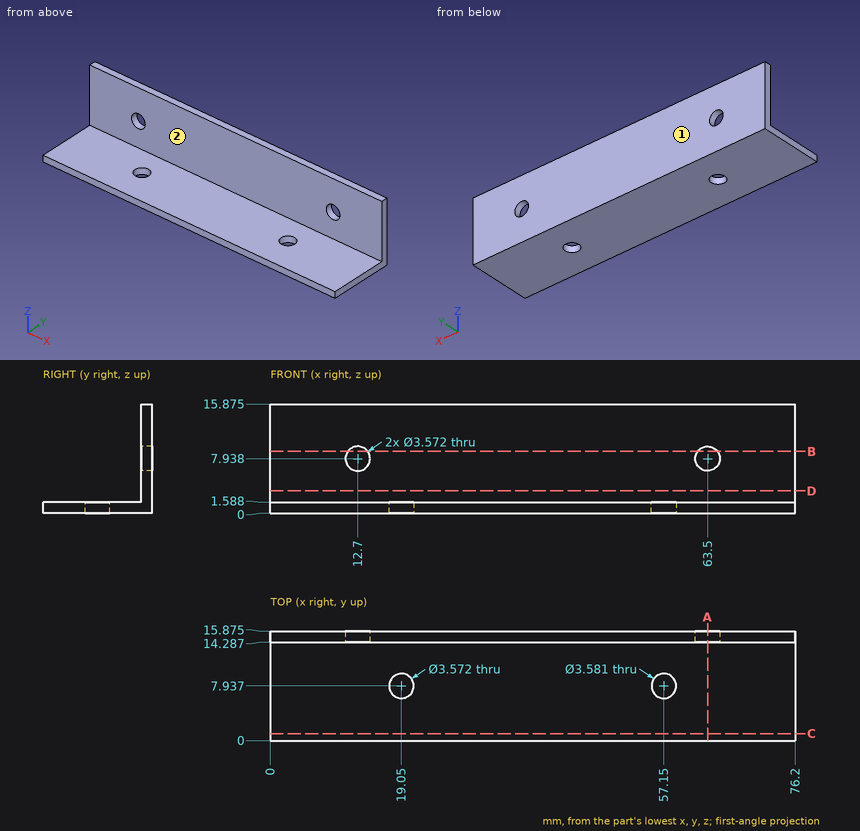
Check sheet for the drawn part. Datum: minimum x, y, z corner. Units: mm. A direction names the side the tool comes from. Coordinates: 2 decimals unless noted, no trailing zeros. Order: outer loops, then holes, each group sorted by start corner. A loop starts at its lowest first (then second) coordinate and runs counter-clockwise, first axis right, second up. Notation, with made-up numbers: M 55.25,-10.75 L 74.25,-10.75 A19 ccw 74.25,10.25 Z; hole C -20,12 d5. An arc over 180 degrees is marked long. One line per item, written item: value. Start each with the question number.
Item 1: Gauge pin test, flat ends, axial feed: pin 1 (1 mm diameter, centred on y = 10.5, z = 3, fed in from -X); pin 2 (8 mm diameter, centred on x = 46, y = 8.5, fed in from -Z); pin 3 (5.5 mm diameter, centred on x = 57.15, y = 7.94, fed in from +Z); pin 4 (4 mm diameter, centred on x = 12.7, z = 7.94, fed in from -Y). Record the tip position at first contact, or that the pin passes through.
Item 2: Access from +Z, -Z, +X, -X, +Y, -Y to the whole of each face (thin tool, end or side, straight path). Record for the marked faces 1 and 2.
Item 3: Sectioned sample at D-D (z = 3.25). Enter the section's corners in (x, y) (1 decimal), then the cut area to 3 significant figures.
Item 4: Scan lines: probe 1 along X at (y, z) = (15, 8) (1 decimal); probe 2 along Z at (x, y) = (63.5, 14.8) (1 decimal). Record each from-to range of solid material in increasing order.
Item 5: Sectioned sample at B-B (z = 9). Enter the section's corners in (x, y) (1 decimal), then the cut area to 3 significant figures.
Item 6: Sectioned sample at A-A (x = 63.5). Enter the section's corners in (y, z) (1 decimal).
Item 7: Sectioned sample at C-C (y = 1). Enter the section's corners in (x, z), then the cut area to 3 significant figures.
Conclusion:
1. pin 1: passes through
1. pin 2: stops at z = 0
1. pin 3: stops at z = 1.59
1. pin 4: stops at y = 14.29
2. face 1: +Z, -Z, +X, -X, +Y
2. face 2: +Z, +X, -X, -Y
3. outline: M 0,14.3 L 76.2,14.3 L 76.2,15.9 L 0,15.9 Z
3. area: 121 mm^2
4. probe 1: x = 0 to 10.9, 14.5 to 61.7, 65.3 to 76.2
4. probe 2: z = 0 to 6.2, 9.7 to 15.9
5. outline: M 0,14.3 L 11.3,14.3 L 11.3,15.9 L 0,15.9 Z; M 14.1,14.3 L 62.1,14.3 L 62.1,15.9 L 14.1,15.9 Z; M 64.9,14.3 L 76.2,14.3 L 76.2,15.9 L 64.9,15.9 Z
5. area: 112 mm^2
6. outline: M 0,0 L 15.9,0 L 15.9,6.2 L 14.3,6.2 L 14.3,1.6 L 0,1.6 Z; M 14.3,9.7 L 15.9,9.7 L 15.9,15.9 L 14.3,15.9 Z
7. outline: M 0,0 L 76.2,0 L 76.2,1.59 L 0,1.59 Z
7. area: 121 mm^2
